Geometry check sheet. Reference: the model listing, model coordinates, mm. Face numbers are marked on the shaded views. A direction names the side the tool comes from. Round coordinates to 2 decimals unless told otherwise and drop trailing zeros. Order: outer loops, then holes, each group sorted by start corner. A loop starts at its lowest first (then second) coordinate and runs counter-clockwise, first axis right, second up.
(1) Set-up check for the marked faces 1 and 2: record each of +Z, -Z, +X, -X, +Y, -Y from which the full face is reachable in a straight line by a thin tool's end or side.
(2) Gauge pin test, flat ends, axial feed: P1, Ø4, axis at y = 14, z = 20, coming from the -X side; P2, Ø2, axis at y = 27.5, z = 5.5, coming from the +X side; P3, Ø5, axis at y = 59.5, z = 15.5, coming from the +X side. Record the tip position at first contact, or that the pin passes through.
(3) Cross-section at A-A on z = 15. Enter the section's corners in (x, y).
(4) Cross-section at C-C on z = -15. Enter the section's corners in (x, y).
(5) Draft check along Y on the marked faces 3, 4 and 5. Enter one of: pulls with the +Y half, pulls with the -Y half, needs draft (parallel to the pull), parting line crosses it, or undercut.
(6) Cross-section at B-B on z = 2.5. Enter the section's corners in (x, y), and give its area (3 significant figures).
(7) Thickness scan on L1, parallel to Z at x = -12.5, y = 6.5; L2, parallel to Y at x = -7.75, z = 11; L3, parallel to X at y = 20.5, z = 23. Record the ranges inside material, lowest first.
from build123d import *

# Parameters (mm, degrees)
BOSS_EXTRUDE1_DEPTH            = 37.5
SKETCH2_W                      = 11
SKETCH2_H                      = 69
CUT_EXTRUDE1_DEPTH             = 67
CUT_EXTRUDE2_REACH             = 94.575
CUT_EXTRUDE2_DIRECTION_2_REACH = 94.575
M5_CLEARANCE_SLOT1_DEPTH       = 3
M5_CLEARANCE_HOLE1_D           = 5.5
CHAMFER1_SIZE                  = 35
CHAMFER1_SIZE2                 = 9.378221735
FILLET1_R                      = 5
FILLET2_R                      = 1


# Read off the part's stored shape, not the designer's step: M5 Clearance Slot1
with BuildPart() as part:
    # Sketch1 → Boss-Extrude1 (new, symmetric)
    with BuildSketch(Plane.XY):
        Polygon((-13.05711135, 70), (-25.4, 0), (0, 0), (0, 70), align=None)
    extrude(amount=BOSS_EXTRUDE1_DEPTH, both=True)

    # Sketch2 → Cut-Extrude1 (cut)
    with BuildSketch(Plane(origin=(0, 70, 0), x_dir=(1, 0, 0), z_dir=(0, 1, 0))):
        with Locations((-5.5, 0)):
            Rectangle(SKETCH2_W, SKETCH2_H)
    extrude(amount=-CUT_EXTRUDE1_DEPTH, mode=Mode.SUBTRACT)

    # Cut-Extrude2: up to this face of the body (flat: up to its plane)
    cut_extrude2_end = Plane(part.part.faces().sort_by_distance((-5.5, 36.5, 34.5))[0])
    # Sketch6 → Cut-Extrude2 (cut, up to the picked face)
    with BuildSketch(Plane.XY.offset(17.5), mode=Mode.PRIVATE) as cut_extrude2_sk1:
        Polygon((-11, 70), (-22.697983939, 3), (-11, 3), align=None)
    cut_extrude2_tool1 = split(extrude(cut_extrude2_sk1.sketch, amount=CUT_EXTRUDE2_REACH, mode=Mode.PRIVATE), bisect_by=cut_extrude2_end, keep=Keep.BOTH, mode=Mode.PRIVATE)
    add(cut_extrude2_tool1.solids().sort_by(Axis((-14.899328, 25.333333, 17.5), (0, 0, 1)))[0], mode=Mode.SUBTRACT)

    # Cut-Extrude2 direction 2: up to this face of the body (flat: up to its plane)
    cut_extrude2_direction_2_end = Plane(part.part.faces().sort_by_distance((-5.5, 36.5, -34.5))[0])
    # Sketch6 → Cut-Extrude2 direction 2 (cut, up to the picked face)
    with BuildSketch(Plane.XY.offset(17.5), mode=Mode.PRIVATE) as cut_extrude2_direction_2_sk1:
        Polygon((-11, 70), (-22.697983939, 3), (-11, 3), align=None)
    cut_extrude2_direction_2_tool1 = split(extrude(cut_extrude2_direction_2_sk1.sketch, amount=-CUT_EXTRUDE2_DIRECTION_2_REACH, mode=Mode.PRIVATE), bisect_by=cut_extrude2_direction_2_end, keep=Keep.BOTH, mode=Mode.PRIVATE)
    add(cut_extrude2_direction_2_tool1.solids().sort_by(Axis((-14.899328, 25.333333, 17.5), (0, 0, -1)))[0], mode=Mode.SUBTRACT)

    # M5 Clearance Slot1 outline → M5 Clearance Slot1 (cut)
    with BuildSketch(Plane(origin=(0, 0, 0), x_dir=(1, 0, 0), z_dir=(0, 1, 0))):
        with BuildLine():
            Line((-9, 12.25), (-6, 12.25))
            ThreePointArc((-6, 12.25), (-3.25, 15), (-6, 17.75))
            Line((-6, 17.75), (-9, 17.75))
            ThreePointArc((-9, 17.75), (-11.75, 15), (-9, 12.25))
        make_face()
        with BuildLine():
            Line((-9, -17.75), (-6, -17.75))
            ThreePointArc((-6, -17.75), (-3.25, -15), (-6, -12.25))
            Line((-6, -12.25), (-9, -12.25))
            ThreePointArc((-9, -12.25), (-11.75, -15), (-9, -17.75))
        make_face()
    extrude(amount=M5_CLEARANCE_SLOT1_DEPTH, mode=Mode.SUBTRACT)

    # M5 Clearance Hole1 (through all)
    with Locations(Plane(origin=(-22.534821987, 3.934507249, 0), x_dir=(0, 0, -1), z_dir=(0.985097838962238, -0.17199490594761452, 0))):
        with Locations((-15, 52.064904762), (15, 27.064904762)):
            Hole(M5_CLEARANCE_HOLE1_D / 2)

    # Chamfer1
    chamfer1_edges = [part.edges().sort_by_distance(p)[0] for p in [
        (0, 70, -36),
        (0, 70, 36),
    ]]
    chamfer1_side = [part.faces().sort_by_distance(p)[0] for p in [
        (0, 1.025914226, 0),
    ]]
    chamfer(chamfer1_edges, length=CHAMFER1_SIZE, length2=CHAMFER1_SIZE2, reference=chamfer1_side[0])

    # Fillet1
    fillet1_edges = [part.edges().sort_by_distance(p)[0] for p in [
        (-22.697983939, 3, 0),
    ]]
    fillet(fillet1_edges, radius=FILLET1_R)

    # Fillet2
    fillet2_edges = [part.edges().sort_by_distance(p)[0] for p in [
        (-8.374681044, 3, -34.5),
        (-16.337425642, 39.429987265, -34.5),
        (-16.337425642, 39.429987265, 34.5),
        (-20.576885612, 4.782848515, -34.5),
        (-8.374681044, 3, 34.5),
        (-20.576885612, 4.782848515, 34.5),
    ]]
    fillet(fillet2_edges, radius=FILLET2_R)


solid = part.part
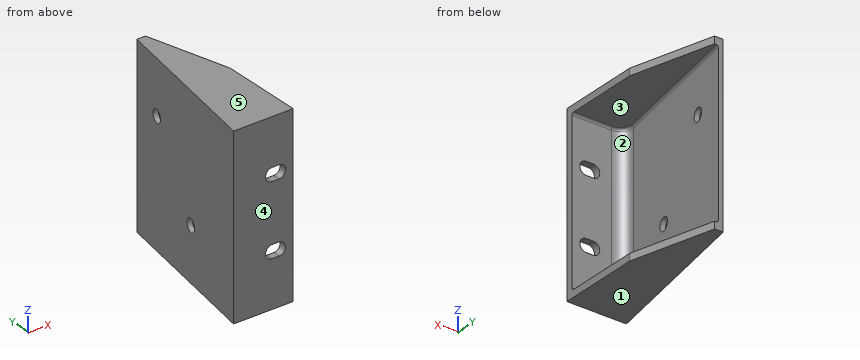
Found:
1. face 1: -Z, +X, -X, +Y, -Y
1. face 2: +X
2. P1: stops at x = -23.28
2. P2: stops at x = -18.25
2. P3: stops at x = -12.4
3. outline: (-25.4, 0) - (-11.75, 0) - (-11.75, 3) - (-16.75, 3) arc R5 cw to (-21.67, 8.86) - (-14.05, 52.51) - (-16.08, 52.87) - close; (-15.12, 58.28) - (-13.11, 57.93) - (-11, 70) - (-13.06, 70) - close; (-3.25, 0) - (0, 0) - (0, 3) - (-3.25, 3) - close
4. outline: (-25.4, 0) - (-11.75, 0) - (-11.75, 3) - (-16.75, 3) arc R5 cw to (-21.67, 8.86) - (-18.35, 27.89) - (-20.42, 28.25) - close; (-19.46, 33.66) - (-17.41, 33.31) - (-11, 70) - (-13.06, 70) - close; (-3.25, 0) - (0, 0) - (0, 3) - (-3.25, 3) - close
5. face 3: undercut
5. face 4: pulls with the -Y half
5. face 5: needs draft
6. outline: (-25.4, 0) - (0, 0) - (0, 3) - (-16.75, 3) arc R5 cw to (-21.67, 8.86) - (-11, 70) - (-13.06, 70) - close
6. area: 225 mm2
7. L1: z = -37.5 to -34.5, 34.5 to 37.5
7. L2: y = 0 to 3
7. L3: x = -21.79 to -19.64
